The model under review builds one solid part; all positions refer to its coordinate system, in mm. Give positions to 0.01 mm unless a question says otherwise; leave off trailing zeros. Use CSV: the item, a comma, the result in double quotes.
Autodesk Inventor part; units mm, degrees
ref_plane "YZ Plane" through (0, 0, 0) normal (1, 0, 0) x (0, 1, 0)
ref_plane "XZ Plane" through (0, 0, 0) normal (0, 1, 0) x (-1, 0, 0)
ref_plane "XY Plane" through (0, 0, 0) normal (0, 0, 1) x (1, 0, 0)
sketch "スケッチ1" plane through (0, 0, 0) normal (0, 0, 1) x (1, 0, 0)
  circle A0 centre (0, 0) radius 40.5
  circle A1 centre (0, 440) radius 40.5
  line L0 (-40.5, 0) -> (-40.5, 440)
  line L1 (40.5, 440) -> (40.5, 0)
  dimension "d0" = 81
  dimension "d1" = 81
  dimension "d2" = 440
extrude "プレート1" add sketch "スケッチ1" along normal blind 2
sketch "スケッチ4" plane through (0, 0, 0) normal (0, 0, -1) x (-1, 0, 0)
  circle A0 centre (0, 0) radius 28
  dimension "d28" = 56
extrude "押し出し1" cut sketch "スケッチ4" against normal blind 10
sketch "スケッチ5" plane through (0, 0, 0) normal (0, 0, -1) x (-1, 0, 0)
  circle A0 centre (0, 0) radius 32
  point P0 (0, 32)
  point P1 (-27.7128, 16)
  point P2 (-27.7128, -16)
  point P3 (0, -32)
  point P4 (27.7128, -16)
  point P5 (27.7128, 16)
  dimension "d31" = 64
  dimension "d34" = 360
hole "穴3" at (0, 32, 0) at (27.7128, 16, 0) at (27.7128, -16, 0) at (0, -32, 0) at (-27.7128, -16, 0) at (-27.7128, 16, 0) direction (0, 0, 1) diameter 4.5 end through all
sketch "スケッチ6" plane through (0, 0, 2) normal (0, 0, 1) x (1, 0, 0)
  arc A0 (40.5, 440) -> (-40.5, 440) centre (0, 440) ccw
  circle A1 centre (0, 440) radius 32.5
  point P0 (0, 0)
  dimension "d43" = 65
extrude "押し出し2" cut sketch "スケッチ6" against normal blind 10
sketch "スケッチ9" plane through (0, 0, 2) normal (0, 0, 1) x (1, 0, 0)
  arc A0 (40.5, 440) -> (-40.5, 440) centre (0, 440) ccw
  circle A1 centre (0, 440) radius 36.5
  point P0 (0, 0)
  point P1 (0, 476.5)
  point P2 (-31.6099, 458.25)
  point P3 (-31.6099, 421.75)
  point P4 (0, 403.5)
  point P5 (31.6099, 421.75)
  point P6 (31.6099, 458.25)
  dimension "d58" = 73
  dimension "d61" = 360
hole "穴5" at (0, 476.5, 2) at (-31.6099, 458.25, 2) at (-31.6099, 421.75, 2) at (0, 403.5, 2) at (31.6099, 421.75, 2) at (31.6099, 458.25, 2) direction (0, 0, -1) diameter 3.2 end through all
sketch "スケッチ16" plane through (0, 0, 2) normal (0, 0, 1) x (1, 0, 0)
  circle A0 centre (0, 355.2097) radius 4
  arc A1 (40.5, 440) -> (-40.5, 440) centre (0, 440) ccw
  circle A2 centre (0, 440) radius 25
  line L0 (-23.4923, 431.4495) -> (4.1883, 355.3977)
  line L1 (0, 603.9) -> (0, -147.9)
  point P0 (0, 0)
  dimension "d154" = 50
  dimension "d135" = 8
  dimension "d136" = 0
  dimension "d137" = 160
hole "穴11" at (0, 355.2097, 2) direction (0, 0, -1) diameter 4.5 end through all
sketch "スケッチ17" plane through (0, 0, 2) normal (0, 0, 1) x (1, 0, 0)
  circle A0 centre (0, 0) radius 44
  point P0 (-4, 72)
  dimension "d145" = 88
  dimension "d177" = 72
  dimension "d178" = 4
hole "穴12" at (-4, 72, 2) direction (0, 0, -1) diameter 4.3 end through all
sketch "スケッチ18" plane through (0, 0, 0) normal (0, 0, -1) x (-1, 0, 0)
  line L0 (-9, 41) -> (9, 41)
  line L1 (9, 41) -> (9, 56)
  line L2 (9, 56) -> (-9, 56)
  line L3 (-9, 56) -> (-9, 41)
  line L4 (-9, 41) -> (9, 56) construction
  line L5 (9, 41) -> (-9, 56) construction
  arc A0 (40.5, 440) -> (-40.5, 440) centre (0, 440) ccw
  point P0 (0, 0)
  point P1 (0, 48.5)
  point P2 (0, 48.5)
  dimension "d157" = 18
  dimension "d158" = 15
  dimension "d183" = 41
extrude "押し出し4" cut sketch "スケッチ18" against normal blind 10
fillet "コーナーR2" radius 2 4 edges at (-9, 56, 1) (9, 56, 1) (9, 41, 1) (-9, 41, 1)
sketch "スケッチ19" plane through (0, 0, 2) normal (0, 0, 1) x (1, 0, 0)
  line L0 (21, 72) -> (-4, 72) construction
  line L1 (21, 69.85) -> (-4, 69.85)
  line L2 (-4, 74.15) -> (21, 74.15)
  arc A0 (21, 69.85) -> (21, 74.15) centre (21, 72) ccw
  arc A1 (-4, 74.15) -> (-4, 69.85) centre (-4, 72) ccw
  circle A2 centre (-4, 72) radius 2.15
  point P0 (0, 0)
  point P1 (8.5, 72)
  dimension "d182" = 21
extrude "押し出し5" cut sketch "スケッチ19" against normal blind 10
sketch "スケッチ20" plane through (0, 0, 0) normal (0, 0, -1) x (-1, 0, 0)
  point P0 (0, 0)
  point P1 (0, 220)
  dimension "d167" = 220
hole "穴13" at (0, 220, 0) direction (0, 0, 1) diameter 4.5 end through all
equation "\"d41\" = Thickness"
equation "\"d68\" = Thickness"
equation "\"d143\" = Thickness"
equation "\"d152\" = Thickness"
equation "\"d173\" = Thickness"
equation "\"d3\" = Thickness"
equation "\"BendRadius\" = Thickness"
equation "\"BendReliefWidth\" = Thickness"
equation "\"BendReliefDepth\" = 0.5 * Thickness"
equation "\"CornerReliefSize\" = 4 * Thickness"
equation "\"MinimumRemnant\" = 2 * Thickness"
equation "\"TransitionRadius\" = BendRadius"
equation "\"JacobiRadiusSize\" = Thickness"
equation "\"GapSize\" = Thickness"
properties part number "link2-plate2" material "CFRP"
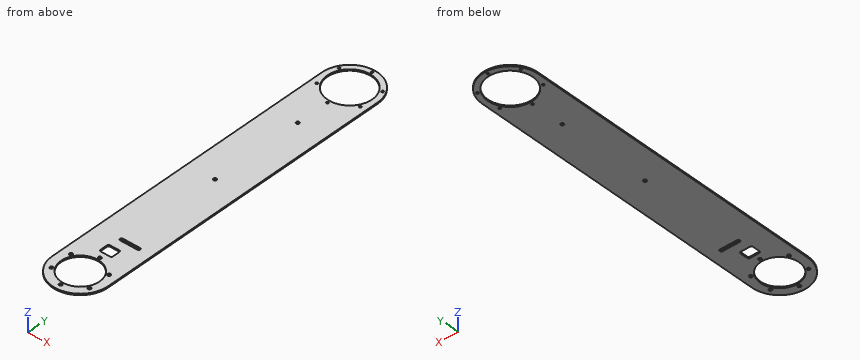
Item 1: Wall thickness on L1, parallel to Y at x = 13, z = 1.7; L2, parallel to Y at x = 6, z = 0.4; L3, parallel to Y at x = 13.5, z = 0.95: over which ranges is each line inside the solid? List them lowest first.
Results list:
L1,"y = -38.36 to -24.8, 24.8 to 69.85, 74.15 to 410.21, 469.79 to 478.36"
L2,"y = -40.05 to -27.35, 27.35 to 41, 56 to 69.85, 74.15 to 408.06, 471.94 to 480.05"
L3,"y = -38.18 to -24.53, 24.53 to 69.85, 74.15 to 410.44, 469.56 to 478.18"
Item 2: Take a section at A-A, the plane z = 1. State how many separate pieces and enclosed holes the cut face has, and give its area (3 significant figures).
Results list:
separate pieces,"1"
enclosed holes,"18"
area,"34,400 mm2"
Item 3: Clearance check with flat-ended pins moving along their axes: pin 1 (0.6 mm diameter, centred on x = 0, z = 1.5, fed in from -Y); pin 2 (2.5 mm diameter, centred on x = -27.71, y = 16, fed in from -Z); pin 3 (0.6 mm diameter, centred on x = 7, z = 1, fed in from -Y). State where each tip first meets the part, or that it passes through.
Results list:
pin 1,"stops at y = -40.5"
pin 2,"passes through"
pin 3,"stops at y = -39.94"
